Input: part model. Units: mm. Frame: model coordinates. Face numbers are marked on the shaded views. A direction names the side the tool comes from. Coordinates: 2 decimals unless noted, no trailing zeros. Write each loop counter-clockwise with the first axis right and the second up, starting at its lowest first coordinate (ties: lowest second). Pieces come first, ordered by that corner, then holes. Notation, with made-up numbers: (58.5, 14.5) - (66.5, 14.5) arc R21 ccw to (66.5, 21.5) - close; hole circle Ø10 at (66, 85). An arc over 180 degrees is marked (long way). Put each result on its own line as item: value. Start each with the question number.
1. Cut plane A-A, the plane x = 68. Return loops of the section in (y, z).
2. Access query for the marked faces 4, 5 and 6. Directions: +Z, -Z, +X, -X, +Y, -Y. A direction counts if a zero-diameter tool reaches every point of the face in a straight line with its end or side. Return the directions, or none.
3. Cut plane D-D, the plane z = -12. Return loops of the section in (x, y).
4. Pull-direction query (X, two-part tool) for the marked faces 1, 2 and 3; classes: released by +X, released by -X, zero draft, split by the parting line, or undercut.
5. Cut plane B-B, the plane y = -38.1. Return loops of the section in (x, z) (1 decimal), and give its area (3 significant figures).
6. Line query: line 1 (Y direction, x = 110, z = 3.5); line 2 (X direction, y = -38.1, z = 2.25); line 3 (X direction, y = -14, z = 6). Output: solid intervals per line, ascending.
7. Pin query (flat end, axial travel): pin 1 (10 mm diameter, centred on x = 101.5, y = -19, fed in from +Z); pin 2 (8 mm diameter, centred on y = -44.5, z = -34, fed in from -X); pin 3 (7 mm diameter, centred on x = 69.596, y = -38.1, fed in from -Z); pin 4 (4 mm diameter, centred on x = 83.5, y = -24.5, fed in from -Z). Return the tip coordinate at first contact, or that it passes through.
8. Cut plane C-C, the plane y = -5. Return loops of the section in (x, z), and give its area (3 significant figures).
from build123d import *

# Parameters (mm, degrees)
F1_DEPTH       = 50.8
F4_D           = 7.9248
F4_DEPTH       = 35.56
F4_CBORE_D     = 12.7
F4_CBORE_DEPTH = 6.096
F4_TIP         = 2.3808501168
F6_DEPTH       = 105.8292752574
F8_DEPTH       = 12.7
F9_DEPTH       = 6.604


with BuildPart() as f1:
    # F0 (on Front) → F1 (new body)
    with BuildSketch(Plane.XZ):
        Polygon((0, 12.7), (0, 0), (85.852, 0), (131.7032699094, -45.8512699094), (140.6835260304, -36.8710137883), (91.1125122421, 12.7), align=None)
    extrude(amount=F1_DEPTH)

    # F4
    with Locations(Plane(origin=(0, 0, 0), x_dir=(1, 0, 0), z_dir=(0, 0, -1))):
        with Locations((15.748, 38.1), (69.596, 38.1), (69.596, 12.7), (15.748, 12.7)):
            CounterBoreHole(F4_D / 2, F4_CBORE_D / 2, F4_CBORE_DEPTH, depth=F4_DEPTH)
            with Locations((0, 0, -(F4_DEPTH + F4_TIP / 2))):  # 118° drill point
                Cone(0, F4_D / 2, F4_TIP, mode=Mode.SUBTRACT)

    # F5 (on face) → F6 (cut, through all)
    with BuildSketch(Plane(origin=(51.9062561211, 0, 51.9062561211), x_dir=(0.7071067812, 0, -0.7071067812), z_dir=(0.7071067812, 0, 0.7071067812))):
        with BuildLine():
            ThreePointArc((125.5500191363, -25.4), (123.9340255134, -38.4929222795), (119.183037491, -50.8))
            Line((119.183037491, -50.8), (125.5500191363, -50.8))
            Line((125.5500191363, -50.8), (125.5500191363, -25.4))
        make_face()
        with BuildLine():
            ThreePointArc((119.183037491, 0), (123.9340255134, -12.3070777205), (125.5500191363, -25.4))
            Line((125.5500191363, -25.4), (125.5500191363, 0))
            Line((125.5500191363, 0), (119.183037491, 0))
        make_face()
    extrude(amount=-F6_DEPTH, mode=Mode.SUBTRACT)

    # F7 (on face) → F8 (join)
    with BuildSketch(Plane(origin=(51.9062561211, 0, 51.9062561211), x_dir=(0.7071067812, 0, -0.7071067812), z_dir=(0.7071067812, 0, 0.7071067812))):
        with BuildLine():
            Line((71.7020191363, -41.148), (71.7020191363, -50.8))
            Line((71.7020191363, -50.8), (119.183037491, -50.8))
            ThreePointArc((119.183037491, -50.8), (121.4241681108, -46.0715990033), (123.1957818654, -41.148))
            Line((123.1957818654, -41.148), (71.7020191363, -41.148))
        make_face()
        with BuildLine():
            Line((119.183037491, 0), (71.7020191363, 0))
            Line((71.7020191363, 0), (71.7020191363, -9.652))
            Line((71.7020191363, -9.652), (123.1957818654, -9.652))
            ThreePointArc((123.1957818654, -9.652), (121.4241681108, -4.7284009967), (119.183037491, 0))
        make_face()
        with BuildLine():
            Line((71.7020191363, -35.052), (71.7020191363, -41.148))
            Line((71.7020191363, -41.148), (123.1957818654, -41.148))
            ThreePointArc((123.1957818654, -41.148), (124.0257032683, -38.1216029987), (124.6779193174, -35.052))
            Line((124.6779193174, -35.052), (71.7020191363, -35.052))
        make_face()
        with BuildLine():
            Line((71.7020191363, -9.652), (71.7020191363, -15.748))
            Line((71.7020191363, -15.748), (124.6779193174, -15.748))
            ThreePointArc((124.6779193174, -15.748), (124.0257032683, -12.6783970013), (123.1957818654, -9.652))
            Line((123.1957818654, -9.652), (71.7020191363, -9.652))
        make_face()
    extrude(amount=F8_DEPTH)

    # F7 (on face) → F9 (cut)
    with BuildSketch(Plane(origin=(51.9062561211, 0, 51.9062561211), x_dir=(0.7071067812, 0, -0.7071067812), z_dir=(0.7071067812, 0, 0.7071067812))):
        with BuildLine():
            Line((71.7020191363, -35.052), (71.7020191363, -41.148))
            Line((71.7020191363, -41.148), (123.1957818654, -41.148))
            ThreePointArc((123.1957818654, -41.148), (124.0257032683, -38.1216029987), (124.6779193174, -35.052))
            Line((124.6779193174, -35.052), (71.7020191363, -35.052))
        make_face()
        with BuildLine():
            Line((71.7020191363, -9.652), (71.7020191363, -15.748))
            Line((71.7020191363, -15.748), (124.6779193174, -15.748))
            ThreePointArc((124.6779193174, -15.748), (124.0257032683, -12.6783970013), (123.1957818654, -9.652))
            Line((123.1957818654, -9.652), (71.7020191363, -9.652))
        make_face()
    extrude(amount=F9_DEPTH, mode=Mode.SUBTRACT)


solid = f1.part
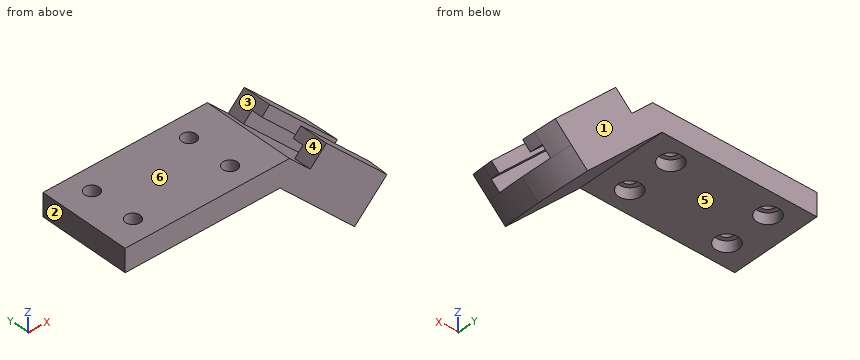
Report:
1. outline: (-50.8, 0) - (-44.25, 0) - (-44.25, 6.1) - (-41.73, 6.1) - (-41.73, 12.7) - (-50.8, 12.7) - close; (-34.47, 6.1) - (-31.95, 6.1) - (-31.95, 0) - (-18.85, 0) - (-18.85, 6.1) - (-16.33, 6.1) - (-16.33, 12.7) - (-34.47, 12.7) - close; (-9.07, 6.1) - (-6.55, 6.1) - (-6.55, 0) - (0, 0) - (0, 12.7) - (-9.07, 12.7) - close
2. face 4: +Z, +Y, -Y
2. face 5: -Z, -X, +Y, -Y
2. face 6: +Z, +X, -X, +Y, -Y
3. outline: (97.85, -50.8) - (133.77, -50.8) - (133.77, -35.05) - (125.15, -35.05) - (125.15, -41.15) - (115.81, -41.15) - (115.81, -9.65) - (125.15, -9.65) - (125.15, -15.75) - (133.77, -15.75) - (133.77, 0) - (97.85, 0) - close
4. face 1: zero draft
4. face 2: released by -X
4. face 3: undercut
5. outline: (0, 0) - (9.4, 0) - (9.4, 6.1) - (11.8, 6.1) - (11.8, 12.7) - (0, 12.7) - close; (19.7, 6.1) - (22.1, 6.1) - (22.1, 0) - (63.2, 0) - (63.2, 6.1) - (65.6, 6.1) - (65.6, 12.7) - (19.7, 12.7) - close; (73.6, 6.1) - (75.9, 6.1) - (75.9, 0) - (85.9, 0) - (130.6, -44.8) - (139.6, -35.8) - (91.1, 12.7) - (73.6, 12.7) - close; (107.3, 5.9) - (144.3, -31.1) - (148.6, -26.8) - (111.6, 10.2) - close
5. area: 2,020 mm^2
6. line 1: y = -50.8 to -35.05, -15.75 to 0
6. line 2: x = 0 to 9.4, 22.1 to 63.25, 75.95 to 101.56, 110.9 to 119.52
6. line 3: x = 0 to 9.53, 21.96 to 63.38, 75.81 to 97.81, 107.4 to 115.77
7. pin 1: stops at z = 7.31
7. pin 2: stops at x = 115.85
7. pin 3: passes through
7. pin 4: stops at z = 0
8. outline: (0, 0) - (85.85, 0) - (128.87, -43.01) - (146.83, -25.05) - (111.59, 10.19) - (102.61, 1.21) - (91.11, 12.7) - (0, 12.7) - close
8. area: 2,560 mm^2
